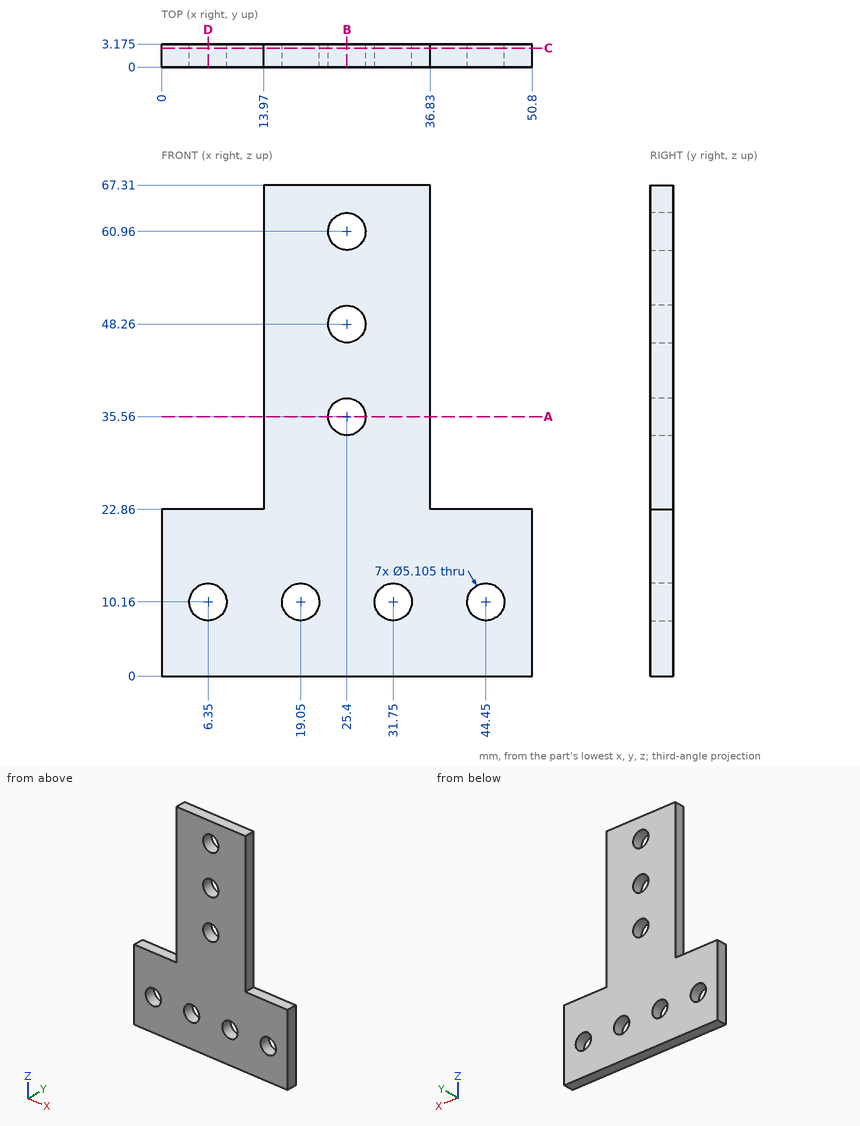
Input: dimensioned drawing with shaded views. Units: mm. Origin: part minimum x, y, z. Coordinates: 2 decimals unless noted, no trailing zeros. Loops run counter-clockwise (first coordinate to the right, second up) from the corner with the lowest first, then second, coordinate; pieces in that order, holes last.
Q1. Contact query for flat-ended pins moving along their axis: pin 1 (6 mm diameter, centred on x = 25.4, z = 35.56, fed in from +Y) (3 decimals); pin 2 (1.6 mm diameter, centred on y = 1.5, z = 36.5, fed in from -X); pin 3 (1 mm diameter, centred on y = 1, z = 51, fed in from +X). Output: stop coordinate, or through.
Results are:
pin 1: stops at y = 3.175
pin 2: stops at x = 13.97
pin 3: stops at x = 36.83
Q2. Line query: line 1 along X through (y, z) = (0.8, 10.16); line 2 along X through (y, z) = (2.2, 35.56); line 3 along X through (y, z) = (1.4, 8). Output: solid intervals per line, ascending.
Results are:
line 1: x = 0 to 3.8, 8.9 to 16.5, 21.6 to 29.2, 34.3 to 41.9, 47 to 50.8
line 2: x = 13.97 to 22.85, 27.95 to 36.83
line 3: x = 0 to 4.99, 7.71 to 17.69, 20.41 to 30.39, 33.11 to 43.09, 45.81 to 50.8
Q3. Section D-D, the plane x = 6.35. Return the cut outline in (y, z) (1 decimal).
Results are:
outline: (0, 0) - (3.2, 0) - (3.2, 7.6) - (0, 7.6) - close; (0, 12.7) - (3.2, 12.7) - (3.2, 22.9) - (0, 22.9) - close
Q4. Section C-C, the plane y = 2.6. Give the number of separate pieces and of enclosed holes in the cut face, and give its area (3 significant figures).
Results are:
separate pieces: 1
enclosed holes: 7
area: 2,030 mm2
Q5. Section B-B, the plane x = 25.4. Return the cut outline in (y, z) (1 decimal).
Results are:
outline: (0, 0) - (3.2, 0) - (3.2, 33) - (0, 33) - close; (0, 38.1) - (3.2, 38.1) - (3.2, 45.7) - (0, 45.7) - close; (0, 50.8) - (3.2, 50.8) - (3.2, 58.4) - (0, 58.4) - close; (0, 63.5) - (3.2, 63.5) - (3.2, 67.3) - (0, 67.3) - close
Q6. Section A-A, the plane z = 35.56. Return the cut outline in (x, y) (1 decimal).
Results are:
outline: (14, 0) - (22.8, 0) - (22.8, 3.2) - (14, 3.2) - close; (28, 0) - (36.8, 0) - (36.8, 3.2) - (28, 3.2) - close
